Check sheet for the drawn part. Datum: minimum x, y, z corner. Units: mm. Coordinates: 2 decimals unless noted, no trailing zeros. Loops run counter-clockwise (first coordinate to the right, second up) from the corner with the lowest first, then second, coordinate; pieces in that order, holes last. Notation, with made-up numbers: M 14,75.5 L 53,75.5 A32 ccw 53,112.5 Z; hole C 19.25,47.5 d11. An arc over 180 degrees is marked long. Answer as CSV lines item,"result". Start each with the question number.
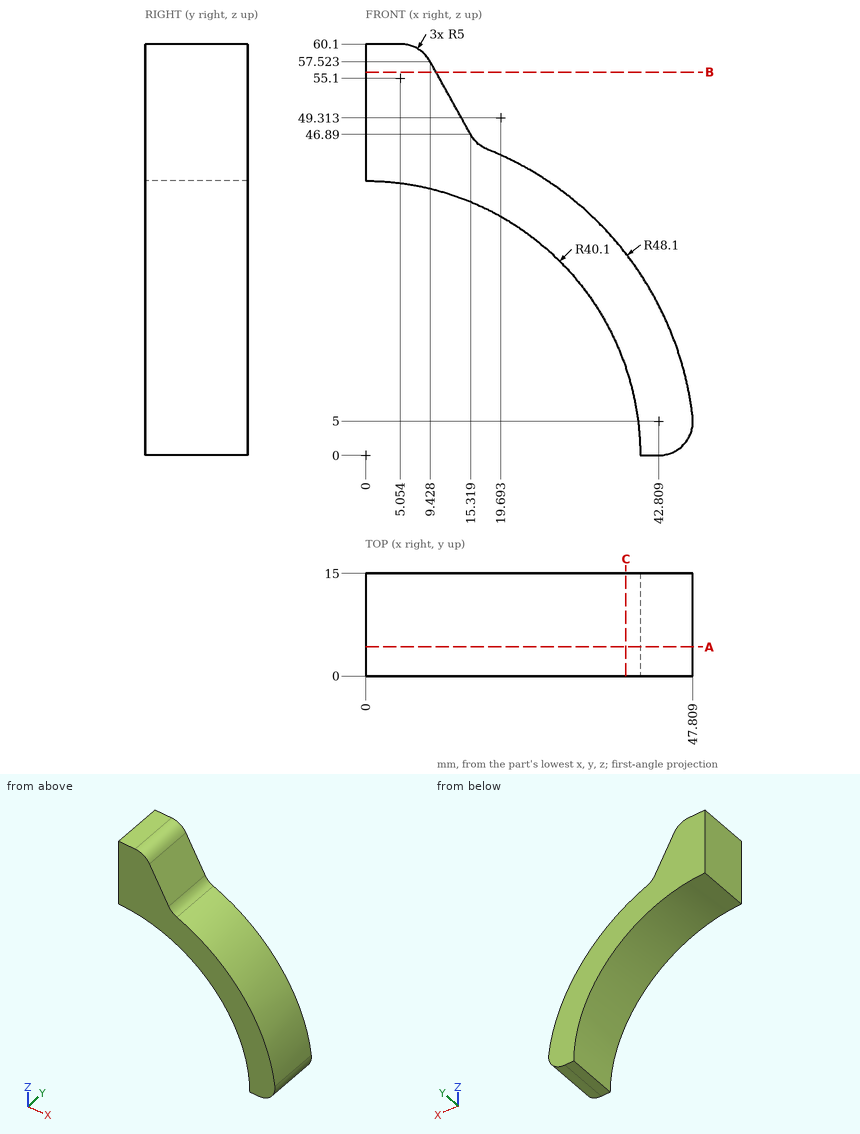
Item 1: Material ranges on line 1 (X direction, y = 1, z = 12.5); line 2 (X direction, y = 7, z = 25) (1 decimal); line 3 (Z direction, x = 15.5, y = 2.75) (1 decimal), recorded low to high. Write a range as from..to.
Item 2: Sectioned sample at A-A, the plane y = 4.25. Record the boundary of the cut face in (x, z) (1 decimal).
Item 3: Go/stop test with flat-tipped pins: pin 1 (2 mm diameter, centred on x = 37, y = 3, fed in from +Z); pin 2 (6 mm diameter, centred on x = 42, y = 12.5, fed in from +Z) (1 decimal); pin 3 (4 mm diameter, centred on y = 10.5, z = 18, fed in from +X). Record where each tip stops, or that it passes through.
Item 4: Sectioned sample at B-B, the plane z = 56. Record the boundary of the cut face in (x, y).
Item 5: Sectioned sample at C-C, the plane x = 38. Record the boundary of the cut face in (y, z).
Reply:
1,line 1,"38.1..46.45"
1,line 2,"31.4..41.1"
1,line 3,"37..46.6"
2,outline,"M 0,40.1 A40.1 cw 40.1,0 L 42.8,0 A5 ccw 47.8,5.6 A48.1 ccw 17.8,44.7 A5 cw 15.3,46.9 L 9.4,57.5 A5 ccw 5.1,60.1 L 0,60.1 Z"
3,pin 1,"z = 31.9"
3,pin 2,"z = 28.2"
3,pin 3,"x = 45.36"
4,outline,"M 0,0 L 10.27,0 L 10.27,15 L 0,15 Z"
5,outline,"M 0,12.81 L 15,12.81 L 15,29.49 L 0,29.49 Z"
